Here's how the part is built. I have some questions about the finished solid (model axes, mm). A direction names the side the tool comes from. Round coordinates to 2 decimals unless told otherwise and drop trailing zeros. Write each loop counter-clockwise with the first axis right and the second up, starting at its lowest first coordinate (ties: lowest second). Pieces come first, ordered by that corner, then holes. Notation, with made-up numbers: (2.5, 67.25) - (7.5, 67.25) arc R14 cw to (7.5, 77.25) - close; hole circle Ø3 at (69, 66.5). An arc over 180 degrees is marked (long way). Write item = value, one per line. Start each with the question number.
Item 1: If we section it at D-D (x = 12): Please give me the cut outline in (y, z).
Item 2: Which directions (+Z, -Z, +X, -X, +Y, -Y) give clear straight access to the entire face, cutting with the end or side of a thin tool? Please do faces 4 (the face through (26, 1, -3.3)), 5 (the face through (28, 1, 3.3)), 6 (the face through (26.9, 3.9, -0.1)), 7 (the face through (0, 4.2, 4)).
Item 3: Thinking about a two-plate mould opening in Z: for faces 1 (the face through (1.09, 4.4, -2.66)), 2 (the face through (10, 2, 3)), 3 (the face through (0, 4.2, -4)), which applies, pulls with the +Z half, pulls with the -Z half, needs draft (parallel to the pull), parting line crosses it, or undercut?
Item 4: If we section it at B-B (x = 23): Please give me the cut outline in (y, z).
Item 5: If we section it at C-C (z = 8): Please give me the cut outline in (x, y).
Item 6: If I drill on line 1 along X through (y, z) = (0.5, -4.5); line 2 along X through (y, z) = (1.9, 0); line 3 along Z through (x, y) = (10.5, 1.45), over which ranges is the centre line in solid material (lowest first)? Write a range as [from, to].
Item 7: For P1, Ø1, axis at y = 1, z = 4, coming from the -X side; P2, Ø1.6, axis at x = 27.5, y = 2, coming from the -Z side; P3, Ø1, axis at y = 2, z = 4.5, coming from the +X side, each with a flat end and sliding along its axis, tell me the tip position at first contact or that it passes through.
```python
from build123d import *

# Parameters (mm, degrees)
SKETCH1_W           = 10
SKETCH1_H           = 6
BOSS_EXTRUDE1_DEPTH = 5
BOSS_EXTRUDE2_DEPTH = 1
BOSS_EXTRUDE3_DEPTH = 7
FILLET1_R           = 5
SKETCH4_W           = 6
SKETCH4_H           = 5
BOSS_EXTRUDE4_DEPTH = 12
SKETCH5_W           = 10
SKETCH5_H           = 5
BOSS_EXTRUDE5_DEPTH = 2
FILLET3_START       = 5.05342
FILLET3_DEPTH       = 13.94658
FILLET3_START_2     = 3
FILLET3_2_DEPTH     = 2.14658
FILLET3_3_DEPTH     = 3
FILLET3_START_3     = -3
FILLET3_4_DEPTH     = 6
BOSS_EXTRUDE6_DEPTH = 16
SKETCH7_R           = 1.6
SKETCH7_W           = 2
SKETCH7_H           = 1
CUT_EXTRUDE1_DEPTH  = 38.027017163
CUT_EXTRUDE6_DEPTH  = 1


with BuildPart() as part:
    # Sketch1 → Boss-Extrude1 (new body)
    with BuildSketch(Plane(origin=(0, 0, 0), x_dir=(1, 0, 0), z_dir=(0, 1, 0))):
        Rectangle(SKETCH1_W, SKETCH1_H)
    extrude(amount=BOSS_EXTRUDE1_DEPTH)

    # Sketch2 → Boss-Extrude2 (add)
    with BuildSketch(Plane.XY.offset(3)):
        with BuildLine():
            Line((5, 0), (-5, 0))
            ThreePointArc((-5, 0), (0, 5), (5, 0))
        make_face()
    boss_extrude2 = extrude(amount=BOSS_EXTRUDE2_DEPTH)

    # Sketch3 → Boss-Extrude3 (add)
    with BuildSketch(Plane.XY.offset(4)):
        with BuildLine():
            Line((-3.9, 0), (3.9, 0))
            ThreePointArc((3.9, 0), (0, 3.9), (-3.9, 0))
        make_face()
    boss_extrude3 = extrude(amount=BOSS_EXTRUDE3_DEPTH)

    # Mirror1: Boss-Extrude2, Boss-Extrude3 across plane
    add(boss_extrude2.mirror(Plane.XY))
    add(boss_extrude3.mirror(Plane.XY))

    # Fillet1
    fillet1_edges = [part.edges().sort_by_distance(p)[0] for p in [
        (-5, 5, 0),
    ]]
    fillet(fillet1_edges, radius=FILLET1_R - 0.0001)  # a hair under: the kernel refuses the full size

    # Sketch4 → Boss-Extrude4 (add)
    with BuildSketch(Plane(origin=(5, 0, 0), x_dir=(0, 0, -1), z_dir=(1, 0, 0))):
        with Locations((0, 2.5)):
            Rectangle(SKETCH4_W, SKETCH4_H)
    extrude(amount=BOSS_EXTRUDE4_DEPTH)

    # Sketch5 → Boss-Extrude5 (add)
    with BuildSketch(Plane(origin=(17, 0, 0), x_dir=(0, 0, -1), z_dir=(1, 0, 0))):
        with Locations((0, 2.5)):
            Rectangle(SKETCH5_W, SKETCH5_H)
    extrude(amount=BOSS_EXTRUDE5_DEPTH)

    # Fillet3: read off the stored shape, not the designer's step
    # Fillet3 outline → Fillet3 (cut)
    with BuildSketch(Plane.YZ.offset(FILLET3_START)):
        with BuildLine():
            ThreePointArc((5, 0), (3.535533906, -3.535533906), (0, -5))
            Line((0, -5), (5, -5))
            Line((5, -5), (5, 0))
        make_face()
        with BuildLine():
            Line((5, 0), (5, 5))
            Line((5, 5), (0, 5))
            ThreePointArc((0, 5), (3.535533906, 3.535533906), (5, 0))
        make_face()
    extrude(amount=FILLET3_DEPTH, mode=Mode.SUBTRACT)

    # Fillet3 2 outline → Fillet3 2 (cut)
    with BuildSketch(Plane.YZ.offset(FILLET3_START_2)):
        with BuildLine():
            Line((5, -3), (5, 0))
            ThreePointArc((5, 0), (4.74341649, -1.58113883), (4, -3))
            Line((4, -3), (5, -3))
        make_face()
        with BuildLine():
            ThreePointArc((4, 3), (4.74341649, 1.58113883), (5, 0))
            Line((5, 0), (5, 3))
            Line((5, 3), (4, 3))
        make_face()
    extrude(amount=FILLET3_2_DEPTH, mode=Mode.SUBTRACT)

    # Fillet3 3 outline → Fillet3 3 (cut)
    with BuildSketch(Plane.YZ):
        with BuildLine():
            Line((5, -3), (5, 0))
            ThreePointArc((5, 0), (4.74341649, -1.58113883), (4, -3))
            Line((4, -3), (5, -3))
        make_face()
        with BuildLine():
            ThreePointArc((4, 3), (4.74341649, 1.58113883), (5, 0))
            Line((5, 0), (5, 3))
            Line((5, 3), (4, 3))
        make_face()
    extrude(amount=FILLET3_3_DEPTH, mode=Mode.SUBTRACT)

    # Fillet3 4 outline → Fillet3 4 (add)
    with BuildSketch(Plane.XY.offset(FILLET3_START_3)):
        with BuildLine():
            ThreePointArc((3, 4), (1.58113883, 4.74341649), (0, 5))
            ThreePointArc((0, 5), (-0.50254481, 4.974680765), (-1, 4.898979485))
            Line((-1, 4.898979485), (-1, 2))
            Line((-1, 2), (4, 2))
            Line((4, 2), (4, 3.25))
            Line((4, 3.25), (3, 4))
        make_face()
    extrude(amount=FILLET3_4_DEPTH)

    # Sketch6 → Boss-Extrude6 (add)
    with BuildSketch(Plane(origin=(19, 0, 0), x_dir=(0, 0, -1), z_dir=(1, 0, 0))):
        with BuildLine():
            Line((-3.9, 0), (3.9, 0))
            ThreePointArc((3.9, 0), (0, 3.9), (-3.9, 0))
        make_face()
    extrude(amount=BOSS_EXTRUDE6_DEPTH)

    # Sketch7 → Cut-Extrude1 (cut, through all)
    with BuildSketch(Plane(origin=(0, 0, 0), x_dir=(-1, 0, 0), z_dir=(0, -1, 0))):
        with Locations(Location((0, 0, 0), (0, 0, 90))):
            Circle(SKETCH7_R)
        with Locations((-27, -3.4)):
            Rectangle(SKETCH7_W, SKETCH7_H)
        with Locations((-27, 3.4)):
            Rectangle(SKETCH7_W, SKETCH7_H)
    extrude(amount=-CUT_EXTRUDE1_DEPTH, mode=Mode.SUBTRACT)

    # Sketch9 → Cut-Extrude6 (cut)
    with BuildSketch(Plane(origin=(0, 5, 0), x_dir=(-1, 0, 0), z_dir=(0, -1, 0))):
        Polygon((-2.85, 1.645448267), (-2.85, -1.645448267), (0, -3.290896534), (2.85, -1.645448267), (2.85, 1.645448267), (0, 3.290896534), align=None)
    extrude(amount=CUT_EXTRUDE6_DEPTH, mode=Mode.SUBTRACT)


solid = part.part
```
Reply:
q1.outline = (0, -3) - (4, -3) arc R5 ccw to (4, 3) - (0, 3) - close
q2.face_4 = -Z, +Y, -Y
q2.face_5 = +Z, +Y, -Y
q2.face_6 = +X, +Y
q2.face_7 = +Z, +Y
q3.face_1 = undercut
q3.face_2 = pulls with the +Z half
q3.face_3 = pulls with the -Z half
q4.outline = (0, -3.9) arc R3.9 ccw to (0, 3.9) - close
q5.outline = (-3.9, 0) - (3.9, 0) arc R3.9 ccw to start
q6.line_1 = [-3.87, 3.87], [17, 19]
q6.line_2 = [-4.62, -1.6], [1.6, 35]
q6.line_3 = [-3, 3]
q7.P1 = -4.97
q7.P2 = -3.65
q7.P3 = 19
